Could you check a few things on this model? Use its own coordinates, in mm. Coordinates: 2 decimals unless noted, no trailing zeros. Loops run counter-clockwise (first coordinate to the right, second up) from the corner with the lowest first, then second, coordinate; pieces in that order, holes last. Notation, with made-up numbers: M -2,-30.75 L 8,-30.75 A10 cw 8,-14.75 Z; hole C 88.25,25.25 d9. An arc over 180 degrees is marked long. Return JSON: item names as keys, results as strings. Group by question number.
from build123d import *

# Parameters (mm, degrees)
BOSS_EXTRUDE1_DEPTH          = 12.7
F_10_0_1935_DIAMETER_HOLE1_D = 4.9149


with BuildPart() as part:
    # Sketch1 → Boss-Extrude1 (new body)
    with BuildSketch(Plane.XY):
        with BuildLine():
            Line((38.1, 33.6042), (38.1, 24.7142))
            Line((38.1, 24.7142), (22.561451151, 24.7142))
            ThreePointArc((22.561451151, 24.7142), (17.4625, 27.2796), (12.363548849, 24.7142))
            Line((12.363548849, 24.7142), (-12.363548849, 24.7142))
            ThreePointArc((-12.363548849, 24.7142), (-17.4625, 27.2796), (-22.561451151, 24.7142))
            Line((-22.561451151, 24.7142), (-38.1, 24.7142))
            Line((-38.1, 24.7142), (-38.1, 33.6042))
            Line((-38.1, 33.6042), (38.1, 33.6042))
        make_face()
    extrude(amount=BOSS_EXTRUDE1_DEPTH)

    # #10 (0.1935) Diameter Hole1 (through all)
    with Locations(Plane(origin=(-30.48, 33.6042, 6.35), x_dir=(0, 0, 1), z_dir=(0, 1, 0))):
        with Locations((0, 0), (0, 30.48), (0, 60.96)):
            Hole(F_10_0_1935_DIAMETER_HOLE1_D / 2)


solid = part.part
(1) We'd pull the mould along Z, two halves only. Please class faces 1 (the face through (1, 29, 12.7)), 2 (the face through (-0.94, 29.1, 4.08)), 3 (the face through (30, 24.714, 9)): +Z half, -Z half, draft (parallel to the pull), parting line (faces both ways), or undercut.
(2) Imagine slicing it at B-B, the plane y = 26.5. Write out the boundary of the cut face in (x, z).
(3) Imagine slicing it at A-A, the plane z = 6.35. Write out the boundary of the cut face in (x, y), then the cut area to 3 significant figures.
(4) Imagine slicing it at D-D, the plane z = 3. Write out the boundary of the cut face in (x, y), then the cut area to 3 significant figures.
(5) If I drill on L1, parallel to X at y = 27.5, z = 6.35; L2, parallel to X at y = 31.5, z = 5.5; L3, parallel to Z at x = 29.5, y = 30.25, over which ranges is the centre line in solid material (lowest first)? Write a range as [from, to].
(6) Imagine slicing it at C-C, the plane x = 30.48. Write out the boundary of the cut face in (y, z).
(7) Will this pin go through, and if not, where does the flat tip stop? P1, Ø6.5, axis at x = 0, z = 6.35, coming from the +Y side.
Checks:
{
 "1": {"face 1": "+Z half", "face 2": "undercut", "face 3": "draft"},
 "2": {"outline": "M -38.1,0 L -20.51,0 L -20.51,12.7 L -38.1,12.7 Z; M -14.41,0 L 14.41,0 L 14.41,12.7 L -14.41,12.7 Z; M 20.51,0 L 38.1,0 L 38.1,12.7 L 20.51,12.7 Z; hole C -30.48,6.35 d4.91; hole C 0,6.35 d4.91; hole C 30.48,6.35 d4.91"},
 "3": {"outline": "M -38.1,24.71 L -32.94,24.71 L -32.94,33.6 L -38.1,33.6 Z; M -28.02,24.71 L -22.56,24.71 A6.35 cw -12.36,24.71 L -2.46,24.71 L -2.46,33.6 L -28.02,33.6 Z; M 2.46,24.71 L 12.36,24.71 A6.35 cw 22.56,24.71 L 28.02,24.71 L 28.02,33.6 L 2.46,33.6 Z; M 32.94,24.71 L 38.1,24.71 L 38.1,33.6 L 32.94,33.6 Z", "area": "510 mm²"},
 "4": {"outline": "M -38.1,24.71 L -22.56,24.71 A6.35 cw -12.36,24.71 L 12.36,24.71 A6.35 cw 22.56,24.71 L 38.1,24.71 L 38.1,33.6 L -38.1,33.6 Z", "area": "641 mm²"},
 "5": {"L1": "[-38.1, -32.94], [-28.02, -2.46], [2.46, 28.02], [32.94, 38.1]", "L2": "[-38.1, -32.79], [-28.17, -2.31], [2.31, 28.17], [32.79, 38.1]", "L3": "[0, 4.1], [8.6, 12.7]"},
 "6": {"outline": "M 24.71,0 L 33.6,0 L 33.6,3.89 L 24.71,3.89 Z; M 24.71,8.81 L 33.6,8.81 L 33.6,12.7 L 24.71,12.7 Z"},
 "7": {"P1": "y = 33.6"}
}
